Source: three-view drawing plus pictorial views. Frame: mm from the lowest corner of the part. A direction names the side the tool comes from. Give positions to 0.01 mm unless a question says otherwise; leave off trailing zeros. Order: outer loops, then holes, each group sorted by start corner. A loop starts at its lowest first (then second) coordinate and runs counter-clockwise, first axis right, second up. Notation, with made-up numbers: (2.5, 21.5) - (54.5, 21.5) arc R20 ccw to (54.5, 51.5) - close; hole circle Ø11 at (-3.75, 88). An arc over 180 degrees is marked (long way). Answer in a Markdown table with one row per item. Add a question column.
1. Contact query for flat-ended pins moving along their axis: pin 1 (2 mm diameter, centred on x = 18, z = 24.5, fed in from -Y); pin 2 (1 mm diameter, centred on y = 3, z = 16, fed in from -X); pin 3 (12 mm diameter, centred on x = 28.5, z = 18.5, fed in from +Y); pin 4 (0.7 mm diameter, centred on x = 6.5, y = 3, fed in from +Z). Output: stop coordinate, or through.
2. Access query for the marked faces 1 and 2. Directions: +Z, -Z, +X, -X, +Y, -Y. A direction counts if a zero-diameter tool reaches every point of the face in a straight line with its end or side. Return the directions, or none.
3. Section query A-A on z = 24.75. Return loops of the section in (x, y), and give its area (3 significant figures).
4. Ray query, line 1 (Z direction, x = 11, y = 6); line 2 (Y direction, x = 6, z = 20.5); line 3 (X direction, y = 3, z = 21). Return the intervals inside material, ascending. Write a range as [from, to].
5. Section query B-B on x = 6. Return loops of the section in (y, z), and give its area (3 significant figures).
6. Section query D-D on z = 2.75. Return loops of the section in (x, y).
7. Section query C-C on y = 2.25. Return loops of the section in (x, z), and give its area (3 significant figures).
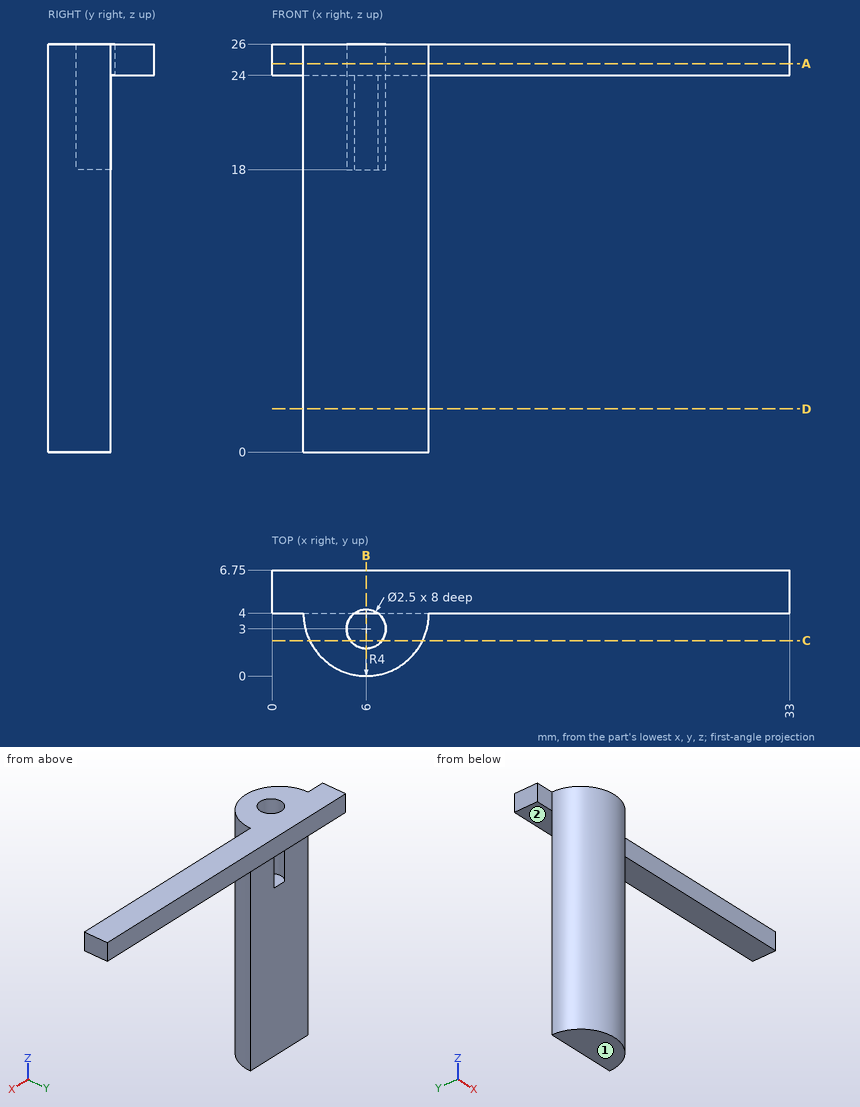
Answer:
| question | item | result |
|---|---|---|
| 1 | pin 1 | stops at y = 4 |
| 1 | pin 2 | stops at x = 2.03 |
| 1 | pin 3 | stops at y = 6.75 |
| 1 | pin 4 | stops at z = 18 |
| 2 | face 1 | -Z, +X, -X, +Y, -Y |
| 2 | face 2 | -Z, +X, -X, +Y |
| 3 | outline | (0, 4) - (2, 4) arc R4 ccw to (10, 4) - (33, 4) - (33, 6.75) - (0, 6.75) - close; hole circle Ø2.5 at (6, 3) |
| 3 | area | 111 mm² |
| 4 | line 1 | z = [24, 26] |
| 4 | line 2 | y = [0, 1.75] |
| 4 | line 3 | x = [2.13, 4.75], [7.25, 9.87] |
| 5 | outline | (0, 0) - (4, 0) - (4, 18) - (1.75, 18) - (1.75, 26) - (0, 26) - close; (4.25, 24) - (6.75, 24) - (6.75, 26) - (4.25, 26) - close |
| 5 | area | 91.0 mm² |
| 6 | outline | (2, 4) arc R4 ccw to (10, 4) - close |
| 7 | outline | (2.4, 0) - (9.6, 0) - (9.6, 26) - (7, 26) - (7, 18) - (5, 18) - (5, 26) - (2.4, 26) - close |
| 7 | area | 171 mm² |
